from build123d import *

# Parameters (mm, degrees)
PROFILE_EXTRUDE_DEPTH                           = 3.175
CSK_FOR_M3_FLAT_HEAD_MACHINE_SCREW1_D           = 3.4
CSK_FOR_M3_FLAT_HEAD_MACHINE_SCREW1_CSINK_D     = 6.3
CSK_FOR_M3_FLAT_HEAD_MACHINE_SCREW1_CSINK_ANGLE = 90
FILM_FEEDER_CLEARANCE_SKETCH_W                  = 46
FILM_FEEDER_CLEARANCE_SKETCH_H                  = 43.35
FILM_FEEDER_CLEARANCE_CUT_DEPTH                 = 4.175
GANTRY_MOUNTING_HOLE_SKETCH_R                   = 1.575
GANTRY_MOUNTING_HOLE_CUT_DEPTH                  = 4.175
ERASER_MOUNTING_HOLE_SKETCH_R                   = 1.575
ERASER_MOUNTING_HOLE_CUT_DEPTH                  = 4.175
FILM_FRICTION_GUIDE_MOUNTING_HOLES_D            = 3.4
FILM_FRICTION_GUIDE_MOUNTING_HOLES_CSINK_D      = 6.3
FILM_FRICTION_GUIDE_MOUNTING_HOLES_CSINK_ANGLE  = 90
BELT_PASSAGEWAY_SKETCH_W                        = 38.1
BELT_PASSAGEWAY_SKETCH_H                        = 12.7
BELT_PASSAGEWAY_CUT_DEPTH                       = 4.175
CSK_FOR_M3_FLAT_HEAD_MACHINE_SCREW3_D           = 3.4
CSK_FOR_M3_FLAT_HEAD_MACHINE_SCREW3_CSINK_D     = 6.3
CSK_FOR_M3_FLAT_HEAD_MACHINE_SCREW3_CSINK_ANGLE = 90


with BuildPart() as part:
    # Profile Sketch → Profile Extrude (new body)
    with BuildSketch(Plane.XY):
        Polygon((73.090000006, 45.35), (129.1, 45.35), (129.1, -45.35), (-129.1, -45.35), (-129.1, 45.35), (-73.090000006, 45.35), (-73.090000006, 97.350000154), (73.090000006, 97.350000154), align=None)
    extrude(amount=PROFILE_EXTRUDE_DEPTH)

    # CSK for M3 Flat Head Machine Screw1 (through all)
    with Locations(Plane(origin=(-121.6, 29.175, 3.175), x_dir=(1, 0, 0), z_dir=(0, 0, 1))):
        with Locations((0, 0), (31, 0), (31, -58.35), (0, -58.35), (212.2, 0), (243.2, 0), (243.2, -58.35), (212.2, -58.35)):
            CounterSinkHole(CSK_FOR_M3_FLAT_HEAD_MACHINE_SCREW1_D / 2, CSK_FOR_M3_FLAT_HEAD_MACHINE_SCREW1_CSINK_D / 2, counter_sink_angle=CSK_FOR_M3_FLAT_HEAD_MACHINE_SCREW1_CSINK_ANGLE)

    # Film Feeder Clearance Sketch → Film Feeder Clearance Cut (cut, through all)
    with BuildSketch(Plane.XY.offset(3.175)):
        with Locations((-106.1, 0)):
            Rectangle(FILM_FEEDER_CLEARANCE_SKETCH_W, FILM_FEEDER_CLEARANCE_SKETCH_H)
        with Locations((106.1, 0)):
            Rectangle(FILM_FEEDER_CLEARANCE_SKETCH_W, FILM_FEEDER_CLEARANCE_SKETCH_H)
    extrude(amount=-FILM_FEEDER_CLEARANCE_CUT_DEPTH, mode=Mode.SUBTRACT)

    # Gantry Mounting Hole Sketch → Gantry Mounting Hole Cut (cut, through all)
    with BuildSketch(Plane.XY.offset(3.175)):
        with Locations((-10.729999994, 89.850000154)):
            Circle(GANTRY_MOUNTING_HOLE_SKETCH_R)
        with Locations((65.470000006, 89.850000154)):
            Circle(GANTRY_MOUNTING_HOLE_SKETCH_R)
        with Locations((65.470000006, 37.850000254)):
            Circle(GANTRY_MOUNTING_HOLE_SKETCH_R)
    extrude(amount=-GANTRY_MOUNTING_HOLE_CUT_DEPTH, mode=Mode.SUBTRACT)

    # Eraser Mounting Hole Sketch → Eraser Mounting Hole Cut (cut, through all)
    with BuildSketch(Plane.XY.offset(3.175)):
        with Locations((-31.230000142, 85.0500001)):
            Circle(ERASER_MOUNTING_HOLE_SKETCH_R)
    extrude(amount=-ERASER_MOUNTING_HOLE_CUT_DEPTH, mode=Mode.SUBTRACT)

    # Film Friction Guide Mounting Holes (through all)
    with Locations(Plane(origin=(-79.925, 12.7, 3.175), x_dir=(1, 0, 0), z_dir=(0, 0, 1))):
        with Locations((0, 0), (0, -25.4), (159.85, 0), (159.85, -25.4)):
            CounterSinkHole(FILM_FRICTION_GUIDE_MOUNTING_HOLES_D / 2, FILM_FRICTION_GUIDE_MOUNTING_HOLES_CSINK_D / 2, counter_sink_angle=FILM_FRICTION_GUIDE_MOUNTING_HOLES_CSINK_ANGLE)

    # Belt Passageway Sketch → Belt Passageway Cut (cut, through all)
    with BuildSketch(Plane.XY.offset(3.175)):
        with Locations((35.470060006, 53.2875)):
            Rectangle(BELT_PASSAGEWAY_SKETCH_W, BELT_PASSAGEWAY_SKETCH_H)
    extrude(amount=-BELT_PASSAGEWAY_CUT_DEPTH, mode=Mode.SUBTRACT)

    # CSK for M3 Flat Head Machine Screw3 (through all)
    with Locations(Plane(origin=(13.245060006, 53.2875, 3.175), x_dir=(1, 0, 0), z_dir=(0, 0, 1))):
        with Locations((0, 0), (44.45, 0)):
            CounterSinkHole(CSK_FOR_M3_FLAT_HEAD_MACHINE_SCREW3_D / 2, CSK_FOR_M3_FLAT_HEAD_MACHINE_SCREW3_CSINK_D / 2, counter_sink_angle=CSK_FOR_M3_FLAT_HEAD_MACHINE_SCREW3_CSINK_ANGLE)


solid = part.part
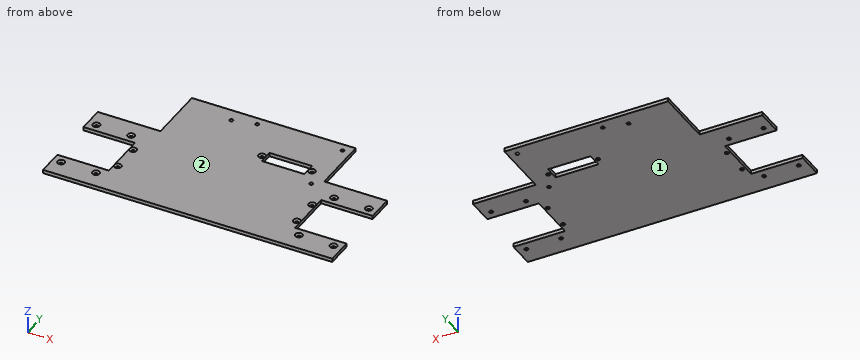
CAD build for the part. Positions are in the model's coordinates, mm. Face numbers are marked on the shaded views. Coordinates: 2 decimals unless noted, no trailing zeros. Loops run counter-clockwise (first coordinate to the right, second up) from the corner with the lowest first, then second, coordinate; pieces in that order, holes last. Notation, with made-up numbers: (-3, -35) - (25, -35) arc R31 ccw to (25, 3) - close; hole circle Ø2 at (10.25, 82.5). An arc over 180 degrees is marked (long way). Use one line per item in the form item = value. Start each with the question number.
1) Two-plate mould, pull along Z, no slides. Class the marked faces 1 and 2: +Z half, -Z half, draft (parallel to the pull), parting line (faces both ways), or undercut.
2) Flat gauge pins, fed straight in: pin 1 (3 mm diameter, centred on x = 57.7, y = 53.29, fed in from -Z); pin 2 (1.6 mm diameter, centred on y = 68.5, z = 2, fed in from +X). Where does each tip first touch, or does it go through?
3) Drill centre lines: L1, parallel to Y at x = -121.6, z = 0.5 (3 decimals); L2, parallel to X at y = 12.7, z = 1.05 (3 decimals); L3, parallel to Y at x = -87, z = 0.25 (3 decimals). Where is each one in solid material? Low to high. Write a range as from..to.
4) Band-saw the part on B-B (y = -4). Give the cut face in (x, z) (3 decimals), and give its area (3 significant figures).
5) Band-saw the part on C-C (z = 0.7). State how many separate pieces and enclosed holes the cut face has, and give its area (3 significant figures).
Check values:
q1.face_1 = -Z half
q1.face_2 = +Z half
q2.pin_1 = through
q2.pin_2 = 73.09
q3.L1 = -45.35..-30.875, -27.475..-21.675, 21.675..27.475, 30.875..45.35
q3.L2 = -83.1..-81.625, -78.225..78.225, 81.625..83.1
q3.L3 = -45.35..-21.675, 21.675..45.35
q4.outline = (-83.1, 0) - (83.1, 0) - (83.1, 3.175) - (-83.1, 3.175) - close
q4.area = 528 mm2
q5.separate_pieces = 1
q5.enclosed_holes = 19
q5.area = 26,400 mm2
